```python
from build123d import *

# Parameters (mm, degrees)
RESSALTO_EXTRUS_O1_DEPTH = 3
SKETCH1_R                = 2.75
CUT_EXTRUDE1_DEPTH       = 10


with BuildPart() as part:
    # Esboço1 → Ressalto-extrusão1 (new body)
    with BuildSketch(Plane(origin=(0, 0, 0), x_dir=(1, 0, 0), z_dir=(0, 1, 0))):
        with BuildLine():
            Line((0, 162.755231864), (0, -162.755231864))
            ThreePointArc((0, -162.755231864), (10.725477972, -190.013301495), (37.150118, -202.653579857))
            Line((37.150118, -202.653579857), (910, -265))
            Line((910, -265), (910, 265))
            Line((910, 265), (37.150118, 202.653579857))
            ThreePointArc((37.150118, 202.653579857), (10.725477972, 190.013301495), (0, 162.755231864))
        make_face()
    extrude(amount=RESSALTO_EXTRUS_O1_DEPTH)

    # Sketch1 → Cut-Extrude1 (cut)
    with BuildSketch(Plane(origin=(0, 3, 0), x_dir=(1, 0, 0), z_dir=(0, 1, 0))):
        with Locations(Location((776.99864992, -221.137424035, 0), (0, 0, 270))):
            Circle(SKETCH1_R)
        with Locations(Location((896.405474423, -229.771178815, 0), (0, 0, 270))):
            Circle(SKETCH1_R)
        with Locations(Location((776.99864992, 216.259876239, 0), (0, 0, 270))):
            Circle(SKETCH1_R)
        with Locations(Location((895.061762745, 227.273960295, 0), (0, 0, 270))):
            Circle(SKETCH1_R)
    extrude(amount=-CUT_EXTRUDE1_DEPTH, mode=Mode.SUBTRACT)


solid = part.part
```
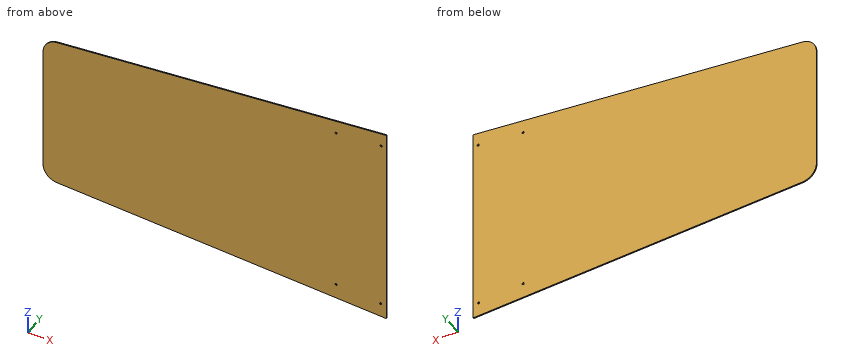
Verification items for the finished model (mm, model axes). Coordinates: 2 decimals unless noted, no trailing zeros. Write each loop counter-clockwise with the first axis right and the second up, starting at its lowest first coordinate (ties: lowest second). Pieces come first, ordered by that corner, then holes. Notation, with made-up numbers: (86.5, 25.5) - (115.5, 25.5) arc R23 ccw to (115.5, 54.5) - close; hole circle Ø9 at (-6, -3). An arc over 180 degrees is marked (long way). One line per question, with ' | ' between items. Start each with the question number.
1. Material ranges on line 1 along Z through (x, y) = (268.5, 2.1); line 2 along Z through (x, y) = (85, 1.5); line 3 along X through (y, z) = (0.35, 194.5), recorded low to high.
2. Section check B-B (x = 476). Enter the section's corners in (y, z).
3. Gauge pin test, flat end, axial feed: P1, Ø3.5, axis at x = 777, z = -216.26, coming from the +Y side. Record the tip position at first contact, or that the pin passes through.
4. Section check A-A (y = 1.2). Enter the section's corners in (x, z).
5. Section check C-C (x = 252.5). Enter the section's corners in (y, z), plus the area to 3 significant figures.
Computed values:
1) line 1: -219.18 to 219.18 | line 2: -206.07 to 206.07 | line 3: 15.66 to 910
2) outline: (0, -234) - (3, -234) - (3, 234) - (0, 234) - close
3) P1: through
4) outline: (0, -162.76) arc R40 ccw to (37.15, -202.65) - (910, -265) - (910, 265) - (37.15, 202.65) arc R40 ccw to (0, 162.76) - close; hole circle Ø5.5 at (777, -216.26); hole circle Ø5.5 at (777, 221.14); hole circle Ø5.5 at (895.06, -227.27); hole circle Ø5.5 at (896.41, 229.77)
5) outline: (0, -218.04) - (3, -218.04) - (3, 218.04) - (0, 218.04) - close | area: 1,310 mm²
